Source: CAD feature listing. Evaluate the final solid. Frame: model axes, mm. Round coordinates to 2 decimals unless told otherwise and drop trailing zeros. Write each loop counter-clockwise with the first axis right and the second up, starting at its lowest first coordinate (ties: lowest second). Pieces come first, ordered by that corner, then holes. Notation, with made-up numbers: M 64.25,-10.5 L 73.25,-10.5 A6 cw 73.25,-5.5 Z; hole C -25.5,71.5 d4. An arc over 180 degrees is marked long. Answer in a Markdown table with one row per item.
Autodesk Inventor part; units mm, degrees
ref_plane "YZ Plane" through (0, 0, 0) normal (1, 0, 0) x (0, 1, 0)
ref_plane "XZ Plane" through (0, 0, 0) normal (0, 1, 0) x (-1, 0, 0)
ref_plane "XY Plane" through (0, 0, 0) normal (0, 0, 1) x (1, 0, 0)
sketch "Sketch1" plane through (0, 0, 0) normal (0, 0, 1) x (1, 0, 0)
  line L0 (-75, 65) -> (75, 65)
  line L1 (75, 65) -> (75, -65)
  line L2 (75, -65) -> (-75, -65)
  line L3 (-75, -65) -> (-75, 65)
  point P0 (0, 0)
  dimension "d0" = 150
  dimension "d1" = 130
  dimension "d2" = 65
  dimension "d3" = 75
extrude "Extrusion1" add sketch "Sketch1" along normal blind 3
sketch "Sketch2" plane through (0, 0, 3) normal (0, 0, 1) x (1, 0, 0)
  circle A0 centre (-60, 40) radius 1.75
  line L0 (75, 65) -> (-75, 65)
  line L1 (-75, 65) -> (-75, -65)
  point P0 (0, 0)
  dimension "d6" = 3.5
  dimension "d15" = 25
  dimension "d16" = 15
extrude "Extrusion2" cut sketch "Sketch2" against normal through all
pattern_linear "Rectangular Pattern1" count 2 spacing 114 along (1, 0, 0) count 2 spacing 80 along (0, -1, 0) of "Extrusion2"
sketch "Sketch3" plane through (0, 0, 3) normal (0, 0, 1) x (1, 0, 0)
  line L0 (75, 65) -> (-75, 65)
  line L1 (-75, 65) -> (-75, -65)
  circle A0 centre (-65, 55) radius 2.75
  point P0 (0, 0)
  dimension "d17" = 5.5
  dimension "d18" = 10
  dimension "d19" = 10
extrude "Extrusion3" cut sketch "Sketch3" against normal through all
pattern_linear "Rectangular Pattern2" count 2 spacing 130 along (1, 0, 0) count 2 spacing 110 along (0, -1, 0) of "Extrusion3"
properties part number "part_plate_rear" material "Polycarbonate, Clear"
Q1. Material intervals for probe 1 along Y at (x, z) = (65, 1.05); probe 2 along Y at (x, z) = (54, 1.3); probe 3 along X at (y, z) = (-55.5, 0.4), sorted ascending.
Solutions:
| item | result |
|---|---|
| probe 1 | y = -65 to -57.75, -52.25 to 52.25, 57.75 to 65 |
| probe 2 | y = -65 to -41.75, -38.25 to 38.25, 41.75 to 65 |
| probe 3 | x = -75 to -67.7, -62.3 to 62.3, 67.7 to 75 |
Q2. Pull-direction query (X, two-part tool) for faces 1 (the cylindrical face through (62.973, -53.141, 1.521)), 2 (the flat face through (75, 1, 1)), 3 (the flat face through (-1, 65, 1)); classes: pulls with the +X half, pulls with the -X half, needs draft (parallel to the pull), parting line crosses it, or undercut.
Solutions:
| item | result |
|---|---|
| face 1 | undercut |
| face 2 | pulls with the +X half |
| face 3 | needs draft |
Q3. Contact query for a flat-ended pin moving along its axis: pin 1 Ø5.5 at (x, y) = (-60, -40) entering from +Z. Output: stop coordinate, or through.
Solutions:
| item | result |
|---|---|
| pin 1 | stops at z = 3 |
Q4. Section A-A (y = 55). Return loops of the section in (x, z), and give its area (3 significant figures).
Solutions:
| item | result |
|---|---|
| outline | M -75,0 L -67.75,0 L -67.75,3 L -75,3 Z; M -62.25,0 L 62.25,0 L 62.25,3 L -62.25,3 Z; M 67.75,0 L 75,0 L 75,3 L 67.75,3 Z |
| area | 417 mm2 |
Q5. Section B-B (x = 54). Return loops of the section in (y, z), and give its area (3 significant figures).
Solutions:
| item | result |
|---|---|
| outline | M -65,0 L -41.75,0 L -41.75,3 L -65,3 Z; M -38.25,0 L 38.25,0 L 38.25,3 L -38.25,3 Z; M 41.75,0 L 65,0 L 65,3 L 41.75,3 Z |
| area | 369 mm2 |
